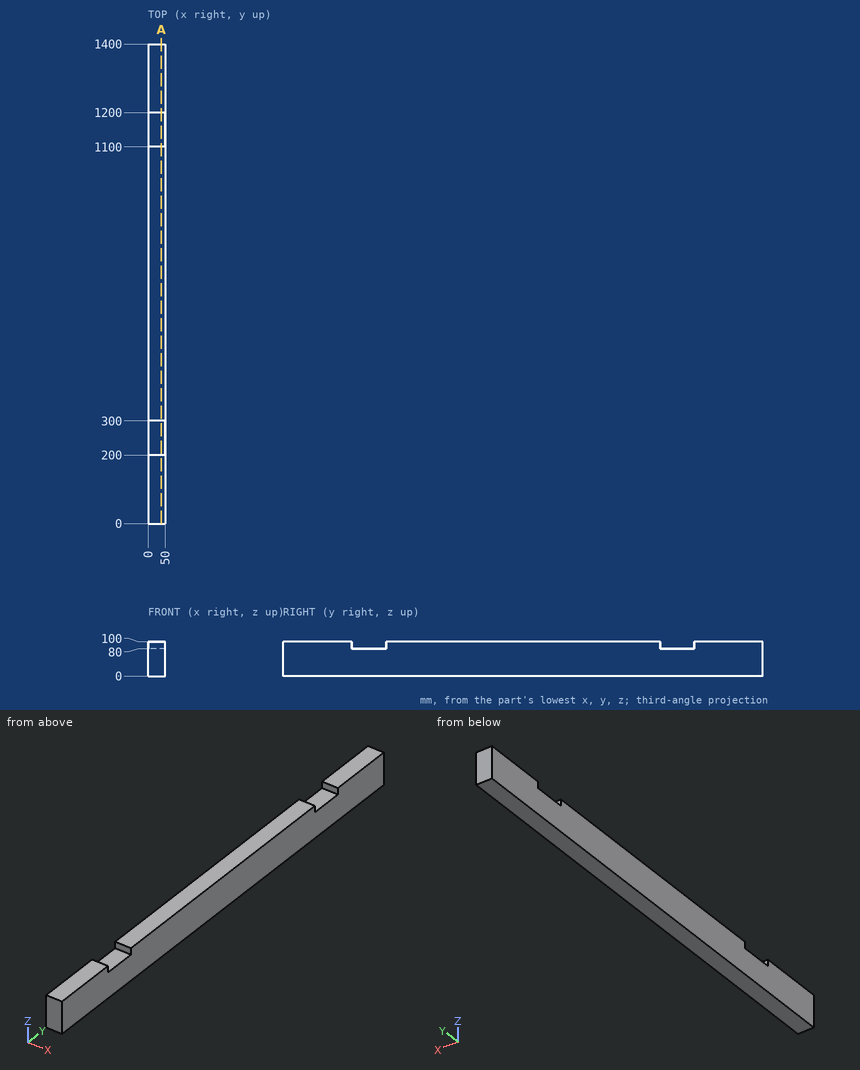
Can you work these out from the drawing? Everything is in mm from the part's minimum corner. Give positions to 0.01 mm unless a question says otherwise; leave off trailing zeros. Order: outer loops, then holes, each group sorted by start corner. A loop starts at its lowest first (then second) coordinate and runs counter-clockwise, first axis right, second up. Notation, with made-up numbers: M 1,24 L 11,24 A17 ccw 11,36 Z; hole C 31,-21 d4. An arc over 180 degrees is marked long. Use a Markdown table: item, result. Add a question column.
Item 1: Suppose I cut it at A-A (x = 38.5). List the corners of the cut face in (y, z) for me, then the cut area to 3 significant figures.
Item 2: If I drill on L1, parallel to Y at x = 14.5, z = 88; L2, parallel to Z at x = 33, y = 271, over which ranges is the centre line in solid material (lowest first)? Write a range as [from, to].
Item 3: Will this pin go through, and if not, where does the flat tip stop? pin 1 (3 mm diameter, centred on y = 172.5, z = 21, fed in from -X).
Answer sheet:
| question | item | result |
|---|---|---|
| 1 | outline | M 0,0 L 1400,0 L 1400,100 L 1200,100 L 1200,80 L 1100,80 L 1100,100 L 300,100 L 300,80 L 200,80 L 200,100 L 0,100 Z |
| 1 | area | 136,000 mm² |
| 2 | L1 | y = [0, 200], [300, 1100], [1200, 1400] |
| 2 | L2 | z = [0, 80] |
| 3 | pin 1 | stops at x = 0 |
